```python
from build123d import *

# Parameters (mm, degrees)
F1_DEPTH  = 3
F3_DEPTH  = 5
F5_DEPTH  = 5
F7_DEPTH  = 5
F9_DEPTH  = 5
F11_R     = 1.5
F12_DEPTH = 55
F14_DEPTH = 100


# Not quite as in the source:
# - a pattern or mirror of a feature is missing from the dataset's text; its kind, count and spacing are read off the source's solid
# - a feature names something its author has since deleted; it is built from what else it names


with BuildPart() as f1:
    # F0 (on Top) → F1 (new body)
    with BuildSketch(Plane.XY):
        Polygon((-20, 62.5), (-25, 62.5), (-25, -62.5), (25, -62.5), (25, 62.5), (20, 62.5), (20, -25.5), (-20, -25.5), align=None)
    extrude(amount=F1_DEPTH)

    # F4 (on face) → F5 (join)
    with BuildSketch(Plane(origin=(-25, 0, 0), x_dir=(0, -1, 0), z_dir=(-1, 0, 0))):
        with BuildLine():
            Line((16.5, 3), (22.5, 3))
            ThreePointArc((22.5, 3), (19.5, 6), (16.5, 3))
        make_face()
    f5 = extrude(amount=-F5_DEPTH)

    # F5_copies: F5 across plane
    add(f5.mirror(Plane(origin=(0, 0, 0), x_dir=(0, 0, 1), z_dir=(1, 0, 0))))

    # F6 (on face) → F7 (join)
    with BuildSketch(Plane(origin=(-25, 0, 0), x_dir=(0, -1, 0), z_dir=(-1, 0, 0))):
        with BuildLine():
            Line((-62.5, 6.1), (-62.5, 3))
            Line((-62.5, 3), (-56.5, 3))
            Line((-56.5, 3), (-56.5, 6.1))
            ThreePointArc((-56.5, 6.1), (-59.5, 3.1), (-62.5, 6.1))
        make_face()
        with BuildLine():
            ThreePointArc((-56.5, 6.1), (-59.5, 9.1), (-62.5, 6.1))
            Line((-62.5, 6.1), (-61, 6.1))
            ThreePointArc((-61, 6.1), (-59.5, 7.6), (-58, 6.1))
            Line((-58, 6.1), (-56.5, 6.1))
        make_face()
        with BuildLine():
            Line((-56.5, 6.1), (-56.5, 3))
            Line((-56.5, 3), (-53.4, 3))
            ThreePointArc((-53.4, 3), (-55.5920310217, 3.9079689783), (-56.5, 6.1))
        make_face()
        with BuildLine():
            Line((-61, 6.1), (-62.5, 6.1))
            ThreePointArc((-62.5, 6.1), (-59.5, 3.1), (-56.5, 6.1))
            Line((-56.5, 6.1), (-58, 6.1))
            ThreePointArc((-58, 6.1), (-59.5, 4.6), (-61, 6.1))
        make_face()
    extrude(amount=-F7_DEPTH)

    # F8 (on face) → F9 (join)
    with BuildSketch(Plane.YZ.offset(25)):
        with BuildLine():
            Line((61, 6.1), (62.5, 6.1))
            ThreePointArc((62.5, 6.1), (59.5, 9.1), (56.5, 6.1))
            Line((56.5, 6.1), (58, 6.1))
            ThreePointArc((58, 6.1), (59.5, 7.6), (61, 6.1))
        make_face()
        with BuildLine():
            Line((56.5, 3), (62.5, 3))
            Line((62.5, 3), (62.5, 6.1))
            ThreePointArc((62.5, 6.1), (59.5, 3.1), (56.5, 6.1))
            Line((56.5, 6.1), (56.5, 3))
        make_face()
        with BuildLine():
            Line((53.4, 3), (56.5, 3))
            Line((56.5, 3), (56.5, 6.1))
            ThreePointArc((56.5, 6.1), (55.5920310217, 3.9079689783), (53.4, 3))
        make_face()
        with BuildLine():
            ThreePointArc((56.5, 6.1), (59.5, 3.1), (62.5, 6.1))
            Line((62.5, 6.1), (61, 6.1))
            ThreePointArc((61, 6.1), (59.5, 4.6), (58, 6.1))
            Line((58, 6.1), (56.5, 6.1))
        make_face()
    extrude(amount=-F9_DEPTH)


with BuildPart() as f3:
    # F2 (on face) → F3 (new body)
    with BuildSketch(Plane.YZ.offset(25)):
        with BuildLine():
            ThreePointArc((-19.5000000146, 0), (-17.3786796616, 0.8786796513), (-16.5, 3))
            Line((-16.5, 3), (-22.5, 3))
            ThreePointArc((-22.5, 3), (-21.6213203487, 0.8786796616), (-19.5000000146, 0))
        make_face()
    extrude(amount=-F3_DEPTH)


with BuildPart() as f1_1:
    add(f1.part)

    # F10: union F3
    add(f3.part)

    # F11 (on face) → F12 (cut)
    with BuildSketch(Plane.YZ.offset(25)):
        with Locations((-19.5, 3)):
            Circle(F11_R)
    extrude(amount=-F12_DEPTH, mode=Mode.SUBTRACT)

    # F13 (on face) → F14 (cut)
    with BuildSketch(Plane.YZ.offset(25)):
        Polygon((-62.5, 3), (-62.5, 0), (-56.5, 3), align=None)
    extrude(amount=-F14_DEPTH, mode=Mode.SUBTRACT)


solid = f1_1.part
```
The model under review builds one solid part; all positions refer to its coordinate system, in mm. A direction names the side the tool comes from. Coordinates: 2 decimals unless noted, no trailing zeros. Loops run counter-clockwise (first coordinate to the right, second up) from the corner with the lowest first, then second, coordinate; pieces in that order, holes last. Notation, with made-up numbers: (-8, 14.25) -> (14, 14.25) arc R12 ccw to (14, 18.25) -> close; hole circle Ø11 at (62, 68). An arc over 180 degrees is marked (long way). Answer as CSV lines item,"result".
Item 1: Take a section at A-A, the plane y = -19.5. State the section outline as (x, z) points, and give its area (3 significant figures).
Results below:
outline,"(-25, 0) -> (-20, 0) -> (-20, 1.5) -> (-25, 1.5) -> close; (-25, 4.5) -> (-20, 4.5) -> (-20, 6) -> (-25, 6) -> close; (20, 0) -> (25, 0) -> (25, 1.5) -> (20, 1.5) -> close; (20, 4.5) -> (25, 4.5) -> (25, 6) -> (20, 6) -> close"
area,"30.0 mm2"
Item 2: Take a section at B-B, the plane y = 50.5. State the section outline as (x, z) points.
Results below:
outline,"(-25, 0) -> (-20, 0) -> (-20, 3) -> (-25, 3) -> close; (20, 0) -> (25, 0) -> (25, 3) -> (20, 3) -> close"
Item 3: Take a section at C-C, the plane x = -7. State the section outline as (y, z) points, and give its area (3 significant figures).
Results below:
outline,"(-62.5, 0) -> (-25.5, 0) -> (-25.5, 3) -> (-56.5, 3) -> close"
area,"102 mm2"
Item 4: Insertion check: pin 1 (5 mm diameter, centred on y = -19.5, z = 3, fed in from -X); pin 2 (3.5 mm diameter, centred on x = -2.5, z = 1, fed in from +Y); pin 3 (4.5 mm diameter, centred on y = 28.5, z = 6, fed in from +X); pin 4 (2.5 mm diameter, centred on x = -23.5, y = 10, fed in from +Z). Each pin has a flat end and moves straight along its axis. Give the tip position at first contact, or say it passes through.
Results below:
pin 1,"stops at x = -25"
pin 2,"stops at y = -25.5"
pin 3,"passes through"
pin 4,"stops at z = 3"
Item 5: Draft analysis for pull direction Z (two halves, no side actions). For faces 4 (the cylindrical face through (-22.535, 55.568, 3.884)), 5 (the cylindrical face through (22.54, 60.93, 5.65)), 6 (the flat face through (-25, 5, 2)), state which applies: +Z half, -Z half, draft (parallel to the pull), parting line (faces both ways), or undercut.
Results below:
face 4,"+Z half"
face 5,"undercut"
face 6,"draft"
Item 6: Machinability: for faces 1 (the flat face through (23, 62.5, 3)), 2 (the flat face through (20, 17.9, 2.6)), 3 (the cylindrical face through (22.535, 55.616, 3.932)), which of the approach directions +Z, -Z, +X, -X, +Y, -Y give a long, thin tool a straight path to every point of the face, cutting with its end or side? Answer none if there is none.
Results below:
face 1,"+Z, -Z, +X, -X, +Y"
face 2,"+Z, -Z, +Y"
face 3,"+Z, +X, -X"
Item 7: For L1, parallel to Y at x = 23.35, z = 6.1; L2, parallel to Z at x = 23.8, y = 59.5; L3, parallel to X at y = 50, z = 2, list the stretches that pass through material, from the lowest coordinate up.
Results below:
L1,"y = 56.5 to 58, 61 to 62.5"
L2,"z = 0 to 4.6, 7.6 to 9.1"
L3,"x = -25 to -20, 20 to 25"
